from build123d import *

# Parameters (mm, degrees)
SKETCH1_R           = 4.15
SKETCH1_W           = 42
SKETCH1_H           = 42
SKETCH1_R_2         = 1.6
SKETCH1_R_3         = 12
BOSS_EXTRUDE1_DEPTH = 2


with BuildPart() as part:
    # Sketch1 → Boss-Extrude1 (new body)
    # profile 1 of 3: a face of its own
    with BuildSketch(Plane(origin=(0, 0, 0), x_dir=(1, 0, 0), z_dir=(0, 1, 0))):
        with BuildLine():
            ThreePointArc((11.023825753, -45.033510687), (9.550490082, -46.826713299), (7.329459099, -47.5))
            Line((7.329459099, -47.5), (-7.329459099, -47.5))
            ThreePointArc((-7.329459099, -47.5), (-9.550490082, -46.826713299), (-11.023825753, -45.033510687))
            Line((-11.023825753, -45.033510687), (-21, -21))
            Line((-21, -21), (21, -21))
            Line((21, -21), (11.023825753, -45.033510687))
        make_face()
        with Locations(Location((-0.154657952, -37.5, 0), (0, 0, 270))):
            Circle(SKETCH1_R, mode=Mode.SUBTRACT)
    # profile 2 of 3: a face of its own
    with BuildSketch(Plane(origin=(0, 0, 0), x_dir=(1, 0, 0), z_dir=(0, 1, 0))):
        Rectangle(SKETCH1_W, SKETCH1_H)
        with Locations(Location((15.5, 15.5, 0), (0, 0, 270))):
            Circle(SKETCH1_R_2, mode=Mode.SUBTRACT)
        with Locations(Location((-15.5, 15.5, 0), (0, 0, 270))):
            Circle(SKETCH1_R_2, mode=Mode.SUBTRACT)
        with Locations(Location((0, 0, 0), (0, 0, 270))):
            Circle(SKETCH1_R_3, mode=Mode.SUBTRACT)
        with Locations(Location((15.5, -15.5, 0), (0, 0, 270))):
            Circle(SKETCH1_R_2, mode=Mode.SUBTRACT)
        with Locations(Location((-15.5, -15.5, 0), (0, 0, 270))):
            Circle(SKETCH1_R_2, mode=Mode.SUBTRACT)
    # profile 3 of 3: a face of its own
    with BuildSketch(Plane(origin=(0, 0, 0), x_dir=(1, 0, 0), z_dir=(0, 1, 0))):
        with BuildLine():
            ThreePointArc((-11.023825753, 45.033510687), (-9.550490082, 46.826713299), (-7.329459099, 47.5))
            Line((-7.329459099, 47.5), (7.329459099, 47.5))
            ThreePointArc((7.329459099, 47.5), (9.550490082, 46.826713299), (11.023825753, 45.033510687))
            Line((11.023825753, 45.033510687), (21, 21))
            Line((21, 21), (-21, 21))
            Line((-21, 21), (-11.023825753, 45.033510687))
        make_face()
        with Locations(Location((-0.154657952, 37.5, 0), (0, 0, 270))):
            Circle(SKETCH1_R, mode=Mode.SUBTRACT)
    extrude(amount=BOSS_EXTRUDE1_DEPTH)


solid = part.part
Check sheet for the modelled part. Datum: model origin and axes. Units: mm. Round coordinates to 2 decimals unless told otherwise and drop trailing zeros. Order: outer loops, then holes, each group sorted by start corner. A loop starts at its lowest first (then second) coordinate and runs counter-clockwise, first axis right, second up. Notation, with made-up numbers: M 85.25,65 L 122.25,65 A29 cw 122.25,89 Z; hole C -21.75,28.25 d10. An arc over 180 degrees is marked long. One line per item, written item: value. Start each with the question number.
1. Scan lines: line 1 along X through (y, z) = (0.95, -15.5); line 2 along Z through (x, y) = (16.5, 1.45); line 3 along Z through (x, y) = (3, 0.7). Record each from-to range of solid material in increasing order.
2. Section check B-B on x = 15.5. Enter the section's corners in (y, z).
3. Release check for a two-part mould opening along X. For faces 1 (the cylindrical face through (-14.42, 0.99, 14.32)), 2 (the flat face through (21, 1, 0)), 3 (the flat face through (-16.1, 1, -32.8)) record: released by +X, released by -X, zero draft, split by the parting line, or undercut.
4. Section check C-C on z = 0. Enter the section's corners in (x, y).
5. Section check A-A on z = 15.5. Enter the section's corners in (x, y), and give its area (3 significant figures).
6. Section check D-D on x = -3. Enter the section's corners in (y, z).
Results found:
1. line 1: -21 to -17.1, -13.9 to 13.9, 17.1 to 21
1. line 2: -31.84 to -16.75, -14.25 to 14.25, 16.75 to 31.84
1. line 3: -47.5 to -40.2, -34.8 to -11.62, 11.62 to 34.8, 40.2 to 47.5
2. outline: M 0,-34.25 L 2,-34.25 L 2,-17.1 L 0,-17.1 Z; M 0,-13.9 L 2,-13.9 L 2,13.9 L 0,13.9 Z; M 0,17.1 L 2,17.1 L 2,34.25 L 0,34.25 Z
3. face 1: undercut
3. face 2: released by +X
3. face 3: released by -X
4. outline: M -21,0 L -12,0 L -12,2 L -21,2 Z; M 12,0 L 21,0 L 21,2 L 12,2 Z
5. outline: M -21,0 L -17.1,0 L -17.1,2 L -21,2 Z; M -13.9,0 L 13.9,0 L 13.9,2 L -13.9,2 Z; M 17.1,0 L 21,0 L 21,2 L 17.1,2 Z
5. area: 71.2 mm^2
6. outline: M 0,-47.5 L 2,-47.5 L 2,-40.52 L 0,-40.52 Z; M 0,-34.48 L 2,-34.48 L 2,-11.62 L 0,-11.62 Z; M 0,11.62 L 2,11.62 L 2,34.48 L 0,34.48 Z; M 0,40.52 L 2,40.52 L 2,47.5 L 0,47.5 Z
